```python
from build123d import *

# Parameters (mm, degrees)
SKETCH1_W           = 25.4
SKETCH1_H           = 12.7
BOSS_EXTRUDE1_DEPTH = 1.5875
SKETCH2_W           = 21.59
SKETCH2_H           = 2.54
SKETCH2_W_2         = 24.13
BOSS_EXTRUDE2_DEPTH = 4.0132


with BuildPart() as part:
    # Sketch1 → Boss-Extrude1 (new body)
    with BuildSketch(Plane(origin=(0, 0, 0), x_dir=(1, 0, 0), z_dir=(0, 1, 0))):
        Rectangle(SKETCH1_W, SKETCH1_H)
    extrude(amount=BOSS_EXTRUDE1_DEPTH)

    # Sketch2 → Boss-Extrude2 (add)
    with BuildSketch(Plane(origin=(0, 1.5875, 0), x_dir=(1, 0, 0), z_dir=(0, 1, 0))):
        with Locations((0, -4.01)):
            Rectangle(SKETCH2_W, SKETCH2_H)
        with Locations((0, -1.37)):
            Rectangle(SKETCH2_W_2, SKETCH2_H)
    boss_extrude2 = extrude(amount=BOSS_EXTRUDE2_DEPTH)

    # Mirror1: Boss-Extrude2 across plane
    add(boss_extrude2.mirror(Plane.XY))


solid = part.part
```
Model file for the job. Use its own axes, mm. A direction names the side the tool comes from. Give positions to 0.01 mm unless a question says otherwise; leave off trailing zeros. Loops run counter-clockwise (first coordinate to the right, second up) from the corner with the lowest first, then second, coordinate; pieces in that order, holes last. Notation, with made-up numbers: M 68.25,-14.5 L 94.25,-14.5 A22 cw 94.25,-4.5 Z; hole C 77,-11 d2. An arc over 180 degrees is marked long. Use one line per item in the form item = value.
Item 1: Slice it at C-C on x = -10.5. List the corners of the cut face in (y, z).
Filled in:
outline = M 0,-6.35 L 1.59,-6.35 L 1.59,-5.28 L 5.6,-5.28 L 5.6,-2.74 L 1.59,-2.74 L 1.59,-2.64 L 5.6,-2.64 L 5.6,-0.1 L 1.59,-0.1 L 1.59,0.1 L 5.6,0.1 L 5.6,2.64 L 1.59,2.64 L 1.59,2.74 L 5.6,2.74 L 5.6,5.28 L 1.59,5.28 L 1.59,6.35 L 0,6.35 Z
Item 2: Slice it at B-B on z = 5. List the corners of the cut face in (x, y) (1 decimal).
Filled in:
outline = M -12.7,0 L 12.7,0 L 12.7,1.6 L 10.8,1.6 L 10.8,5.6 L -10.8,5.6 L -10.8,1.6 L -12.7,1.6 Z
Item 3: Two-plate mould, pull along Z, no slides. Class faces 5 (the flat face through (0, 4, -0.1)), 6 (the flat face through (-12.065, 4, -1)), 7 (the flat face through (0, 1, -6.35)): released by +Z, released by -Z, zero draft, split by the parting line, or undercut.
Filled in:
face_5 = undercut
face_6 = zero draft
face_7 = released by -Z
Item 4: Which spindle directions (+Z, -Z, +X, -X, +Y, -Y) get a long thin tool onto all of the face, cutting with end or side? Do faces 1 (the flat face through (-10.795, 4, 4)), 2 (the flat face through (0, 4, 0.1)), 3 (the flat face through (-12.065, 4, 1)), 4 (the flat face through (10.795, 4, -4)). Say none if no direction does.
Filled in:
face_1 = +Z, -X, +Y
face_2 = +X, -X, +Y
face_3 = +Z, -Z, -X, +Y
face_4 = -Z, +X, +Y
Item 5: Drill centre lines: L1, parallel to Y at x = -11.5, z = 0; L2, parallel to X at y = 3.4, z = -1.5 (3 decimals); L3, parallel to X at y = 4.65, z = 3.5 (3 decimals). Where is each one in solid material? Low to high.
Filled in:
L1 = 0 to 1.59
L2 = -12.065 to 12.065
L3 = -10.795 to 10.795
Item 6: Slice it at A-A on y = 3.5. List the corners of the cut face in (x, z) (3 decimals).
Filled in:
outline = M -12.065,-2.64 L 12.065,-2.64 L 12.065,-0.1 L -12.065,-0.1 Z; M -12.065,0.1 L 12.065,0.1 L 12.065,2.64 L -12.065,2.64 Z; M -10.795,-5.28 L 10.795,-5.28 L 10.795,-2.74 L -10.795,-2.74 Z; M -10.795,2.74 L 10.795,2.74 L 10.795,5.28 L -10.795,5.28 Z
Item 7: Flat gauge pins, fed straight in: pin 1 Ø3 at (y, z) = (4, 4) entering from -X (3 decimals); pin 2 Ø1.2 at (x, y) = (-3, 3) entering from -Z; pin 3 Ø3 at (x, y) = (-5.5, 3) entering from +Z; pin 4 Ø2 at (y, z) = (4, -2) entering from +X (3 decimals). Where does each tip first touch, or does it go through?
Filled in:
pin_1 = -12.065
pin_2 = -5.28
pin_3 = 6.35
pin_4 = 12.065
